Work out the finished part from the listing and answer in its coordinate system (mm). A direction names the side the tool comes from. Round coordinates to 2 decimals unless told otherwise and drop trailing zeros. Write each loop counter-clockwise with the first axis right and the second up, starting at its lowest first coordinate (ties: lowest second). Pieces come first, ordered by that corner, then holes. Notation, with made-up numbers: M -37,5 L -5,5 A29 ccw -5,35 Z; hole C -36.75,64 d6. An arc over 180 degrees is marked long. One line per item, written item: value. Start each with the question number.
Q1. Find section C-C (y = 0.5). Write down the section's boundary in (x, z).
Q2. Find section A-A (z = -79.5). Write down the section's boundary in (x, y), and give its area (3 significant figures).
Q3. A tool of negligible diameter and unlimited length cuts with its end or side. For faces 1 (the flat face through (0, 1, 47)), 2 (the flat face through (8.5, 2, -87)), from which of +Z, -Z, +X, -X, +Y, -Y can it reach the whole face along a straight path? Write none if from no direction.
Q4. The mould has two halves that part along X. Classify faces 3 (the flat face through (-18.5, 1, -26)), 4 (the flat face through (-10, 2, -67.833)), 5 (the flat face through (0, 3, -24)), 6 (the flat face through (18.5, 1, -24)): released by +X, released by -X, zero draft, split by the parting line, or undercut.
Q5. Find section B-B (x = -10). Write down the section's boundary in (y, z), and give its area (3 significant figures).
Q6. Consider probe 1 along X at (y, z) = (2.45, -79.5); probe 2 along X at (y, z) = (2.25, -74); probe 3 along Z at (x, y) = (-10, 2.05). Determine where each line is inside the solid, lowest interval first.
Autodesk Inventor part; units mm, degrees
ref_plane "YZ Plane" through (0, 0, 0) normal (1, 0, 0) x (0, 1, 0)
ref_plane "XZ Plane" through (0, 0, 0) normal (0, 1, 0) x (-1, 0, 0)
ref_plane "XY Plane" through (0, 0, 0) normal (0, 0, 1) x (1, 0, 0)
sketch "Sketch2" plane through (0, 0, 0) normal (0, 1, 0) x (-1, 0, 0)
  line L0 (8.5, 37) -> (-8.5, 37)
  line L1 (-8.5, 37) -> (-8.5, -37)
  line L2 (-8.5, -37) -> (8.5, -37)
  line L3 (8.5, -37) -> (8.5, 37)
  line L4 (8.5, 37) -> (-8.5, -37) construction
  line L5 (-8.5, 37) -> (8.5, -37) construction
  line L6 (18.5, 47) -> (-18.5, 47)
  line L7 (-18.5, 47) -> (-18.5, -47)
  line L8 (-18.5, -47) -> (18.5, -47)
  line L9 (18.5, -47) -> (18.5, 47)
  line L10 (18.5, -47) -> (-18.5, -47)
  line L11 (-18.5, -47) -> (-18.5, -97)
  line L12 (-18.5, -97) -> (18.5, -97)
  line L13 (18.5, -97) -> (18.5, -47)
  point P0 (0, 0)
  dimension "d0" = 17
  dimension "d1" = 74
  dimension "d2" = 10
  dimension "d5" = 50
extrude "Extrusion1" add sketch "Sketch2" along normal blind 3 contours L3 L2 L1 L0 | L9 L8 L7 L6 | L13 L12 L11 L8
sketch "Sketch3" plane through (0, 3, 0) normal (0, 1, 0) x (1, 0, 0)
  line L0 (8.5, 67.8333) -> (8.5, 75.5)
  line L1 (8.5, 67.8333) -> (11.5, 67.8333)
  line L2 (11.5, 75.5) -> (11.5, 67.8333)
  line L3 (8.5, 75.5) -> (11.5, 75.5)
  line L4 (8.5, 83.5) -> (8.5, 91.1667)
  line L5 (8.5, 83.5) -> (11.5, 83.5)
  line L6 (11.5, 91.1667) -> (11.5, 83.5)
  line L7 (8.5, 91.1667) -> (11.5, 91.1667)
  line L8 (-11.5, 83.5) -> (-11.5, 91.1667)
  line L9 (-11.5, 83.5) -> (-8.5, 83.5)
  line L10 (-8.5, 91.1667) -> (-8.5, 83.5)
  line L11 (-11.5, 91.1667) -> (-8.5, 91.1667)
  line L12 (-11.5, 67.8333) -> (-11.5, 75.5)
  line L13 (-11.5, 67.8333) -> (-8.5, 67.8333)
  line L14 (-8.5, 75.5) -> (-8.5, 67.8333)
  line L15 (-11.5, 75.5) -> (-8.5, 75.5)
  line L16 (8.5, 75.5) -> (11.5, 83.5) construction
  line L17 (11.5, 75.5) -> (8.5, 83.5) construction
  line L18 (-8.5, 75.5) -> (-11.5, 83.5) construction
  line L19 (-11.5, 75.5) -> (-8.5, 83.5) construction
  circle A0 centre (-10, 79.5) radius 1.35
  circle A1 centre (10, 79.5) radius 1.35
  point P0 (0, 0)
  dimension "d6" = 2.7
  dimension "d7" = 2.7
extrude "Extrusion2" cut sketch "Sketch3" against normal blind 3
properties part number "bed" material "Acrylic, Clear"
The answers:
1. outline: M -18.5,-97 L 18.5,-97 L 18.5,47 L -18.5,47 Z; hole M -11.5,-91.17 L -8.5,-91.17 L -8.5,-83.5 L -11.5,-83.5 Z; hole M -11.5,-75.5 L -8.5,-75.5 L -8.5,-67.83 L -11.5,-67.83 Z; hole C -10,-79.5 d2.7; hole M 8.5,-91.17 L 11.5,-91.17 L 11.5,-83.5 L 8.5,-83.5 Z; hole M 8.5,-75.5 L 11.5,-75.5 L 11.5,-67.83 L 8.5,-67.83 Z; hole C 10,-79.5 d2.7
2. outline: M -18.5,0 L -11.35,0 L -11.35,3 L -18.5,3 Z; M -8.65,0 L 8.65,0 L 8.65,3 L -8.65,3 Z; M 11.35,0 L 18.5,0 L 18.5,3 L 11.35,3 Z
2. area: 94.8 mm2
3. face 1: +Z, +X, -X, +Y, -Y
3. face 2: +Y, -Y
4. face 3: released by -X
4. face 4: undercut
4. face 5: zero draft
4. face 6: released by +X
5. outline: M 0,-97 L 3,-97 L 3,-91.17 L 0,-91.17 Z; M 0,-83.5 L 3,-83.5 L 3,-80.85 L 0,-80.85 Z; M 0,-78.15 L 3,-78.15 L 3,-75.5 L 0,-75.5 Z; M 0,-67.83 L 3,-67.83 L 3,47 L 0,47 Z
5. area: 378 mm2
6. probe 1: -18.5 to -11.35, -8.65 to 8.65, 11.35 to 18.5
6. probe 2: -18.5 to -11.5, -8.5 to 8.5, 11.5 to 18.5
6. probe 3: -97 to -91.17, -83.5 to -80.85, -78.15 to -75.5, -67.83 to 47
